Autodesk Inventor part; units mm, degrees
ref_plane "YZ Plane" through (0, 0, 0) normal (1, 0, 0) x (0, 1, 0)
ref_plane "XZ Plane" through (0, 0, 0) normal (0, 1, 0) x (-1, 0, 0)
ref_plane "XY Plane" through (0, 0, 0) normal (0, 0, 1) x (1, 0, 0)
sketch "Sketch1" plane through (0, 0, 0) normal (0, 1, 0) x (-1, 0, 0)
  line L0 (0, 0) -> (-6.35, 0)
  line L1 (-6.35, 0) -> (-6.35, -244)
  line L2 (-6.35, -244) -> (0, -244)
  line L3 (0, -244) -> (0, 0)
  dimension "d0" = 6.35
  dimension "d1" = 244
extrude "Extrusion1" add sketch "Sketch1" along normal blind 6.35
sketch "Sketch2" plane through (6.35, 0, 0) normal (1, 0, 0) x (0, 0, -1)
  line L0 (0, 0) -> (244, 0)
  line L1 (0, 0) -> (6.35, 6.35)
  line L2 (0, 6.35) -> (244, 6.35)
  line L3 (0, 0) -> (8.9803, 0) construction
  line L4 (6.35, 6.35) -> (0, 6.35)
  line L5 (0, 6.35) -> (0, 0)
  dimension "d4" = 45
extrude "Extrusion2" cut sketch "Sketch2" against normal blind 10
sketch "Sketch3" plane through (6.35, 0, -244) normal (1, 0, 0) x (0, 0, -1)
  line L0 (0, 0) -> (-6.35, 6.35)
  line L1 (0, 6.35) -> (-237.65, 6.35)
  line L2 (0, 0) -> (8.9803, 0) construction
  line L3 (-6.35, 6.35) -> (0, 6.35)
  line L4 (0, 6.35) -> (0, 0)
  point P0 (-244, 0)
  dimension "d7" = 135
extrude "Extrusion3" cut sketch "Sketch3" against normal blind 10
sketch "Sketch4" plane through (6.35, 0, 0) normal (1, 0, 0) x (0, 0, -1)
  line L0 (0, 0) -> (6.35, 6.35)
  line L1 (244, 0) -> (0, 0)
  line L2 (6.35, 0) -> (12.4246, 0)
  line L3 (237.65, 6.35) -> (6.35, 6.35)
  line L4 (12.4246, 6.35) -> (12.4246, 0)
  line L5 (12.4246, 6.35) -> (6.35, 6.35)
  line L6 (0, 0) -> (6.35, 0)
  line L7 (0, 0) -> (6.35, 6.35)
  dimension "d11" = 6.35
extrude "Extrusion4" cut sketch "Sketch4" against normal blind 10
sketch "Sketch5" plane through (6.35, 0, -12.4246) normal (1, 0, 0) x (0, 0, -1)
  point P0 (-12.4246, 0)
sketch "Sketch6" plane through (6.35, 0, -12.4246) normal (1, 0, 0) x (0, 0, -1)
  line L0 (0, 6.35) -> (0, 0)
  line L1 (0, 0) -> (6.35, 6.35)
  line L2 (225.2254, 6.35) -> (0, 6.35)
  line L3 (0, 0) -> (8.9803, 0) construction
  line L4 (6.35, 6.35) -> (0, 6.35)
  line L5 (231.5754, 0) -> (0, 0)
  line L6 (0, 6.35) -> (0, 0)
  point P0 (-12.4246, 0)
  dimension "d14" = 45
extrude "Extrusion5" cut sketch "Sketch6" against normal blind 10
properties part number "TopTop"
Can you work these out from the model? Positions are in its coordinate system, mm. Give positions to 0.01 mm unless a question says otherwise; leave off trailing zeros. Loops run counter-clockwise (first coordinate to the right, second up) from the corner with the lowest first, then second, coordinate; pieces in that order, holes last. Notation, with made-up numbers: M 6,87 L 43,87 A7 cw 43,91 Z; hole C 46.25,46.25 d6. An arc over 180 degrees is marked long. One line per question, with ' | ' between items. Start each with the question number.
Q1. If we section it at A-A (x = 5.25): Please give me the cut outline in (y, z), plus the area to 3 significant figures.
Q2. For pin 1 Ø1 at (x, z) = (2.5, -206) entering from -Y; pin 2 Ø1 at (x, y) = (3, 2.5) entering from +Z, each with a flat end and sliding along its axis, tell me the tip position at first contact or that it passes through.
Q3. If I drill on line 1 (Z direction, x = 3.5, y = 1.25); line 2 (Z direction, x = 5.75, y = 6.25), over which ranges is the centre line in solid material (lowest first)? Write a range as from..to.
Q4. If we section it at B-B (y = 3.75): Please give me the cut outline in (x, z), plus the area to 3 significant figures.
Computed:
1) outline: M 0,-244 L 6.35,-237.65 L 6.35,-18.77 L 0,-12.42 Z | area: 1,430 mm²
2) pin 1: stops at y = 0 | pin 2: stops at z = -14.42
3) line 1: z = -242.75..-13.67 | line 2: z = -237.75..-18.67
4) outline: M 0,-240.25 L 6.35,-240.25 L 6.35,-16.17 L 0,-16.17 Z | area: 1,420 mm²
